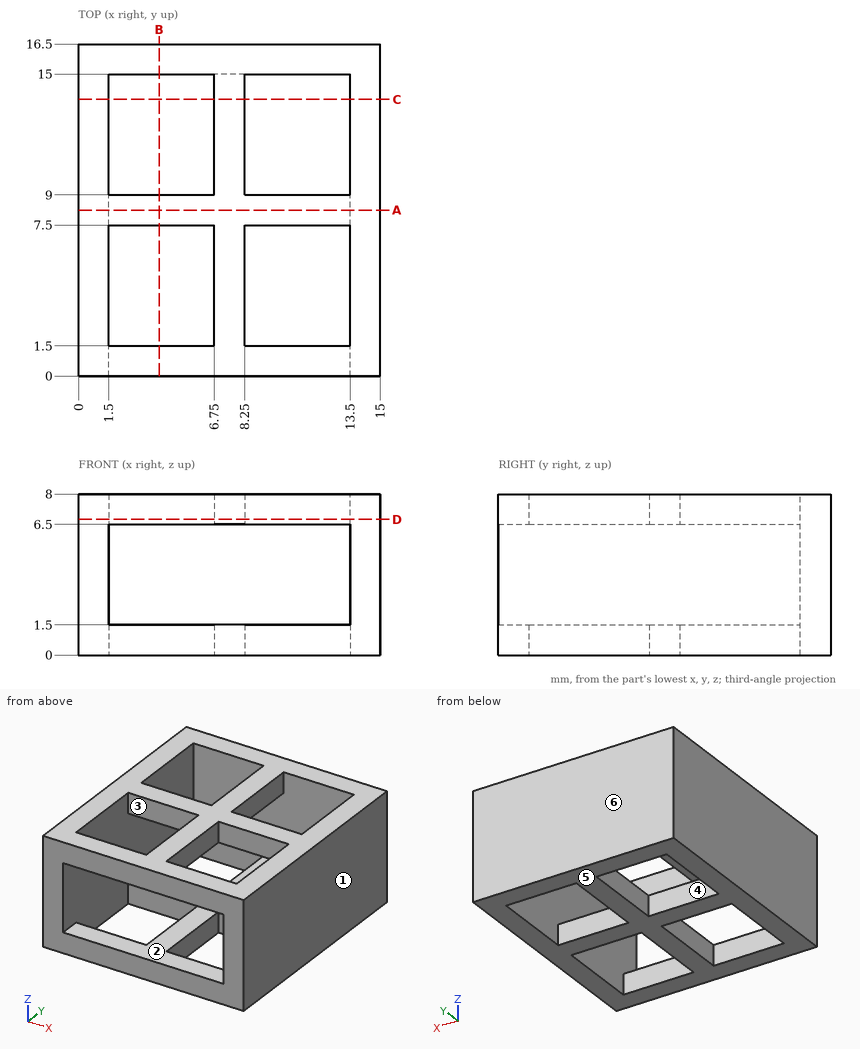
Input: dimensioned drawing with shaded views. Units: mm. Origin: part minimum x, y, z. A direction names the side the tool comes from. Coordinates: 2 decimals unless noted, no trailing zeros. Loops run counter-clockwise (first coordinate to the right, second up) from the corner with the lowest first, then second, coordinate; pieces in that order, holes last. Notation, with made-up numbers: M 63,34.25 L 80,34.25 A30 cw 80,59.25 Z; hole C 44,59 d6. An arc over 180 degrees is marked long. Use a Markdown table: item, result. Add a question column.
1) Section B-B, the plane x = 4. Return the cut outline in (y, z), plus the area to 3 significant figures.
2) Draft query along Y for the marked faces 4, 5 and 6. Return one class per face: +Y half, -Y half, draft (parallel to the pull), parting line (faces both ways), or undercut.
3) Section C-C, the plane y = 13.75. Return the cut outline in (x, z), plus the area to 3 significant figures.
4) Section A-A, the plane y = 8.25. Return the cut outline in (x, z), plus the area to 3 significant figures.
5) Section D-D, the plane z = 6.75. Return the cut outline in (x, y).
6) Line query: L1, parallel to Y at x = 4, z = 0.75; L2, parallel to X at y = 9.25, z = 7.75; L3, parallel to X at y = 9.5, z = 3.5. Output: solid intervals per line, ascending. Write a range as from..to.
7) Pin query (flat end, axial travel): P1, Ø1.2, axis at x = 4.5, z = 0.5, coming from the -Y side. Return the tip coordinate at first contact, or that it passes through.
8) Set-up query: the marked faces 1, 2 and 3. Return all of +Z, -Z, +X, -X, +Y, -Y with unobstructed straight access to the full face (end or side cutting, diameter ignored); none if empty.
Answer below:
| question | item | result |
|---|---|---|
| 1 | outline | M 0,0 L 1.5,0 L 1.5,1.5 L 0,1.5 Z; M 0,6.5 L 1.5,6.5 L 1.5,8 L 0,8 Z; M 7.5,0 L 9,0 L 9,1.5 L 7.5,1.5 Z; M 7.5,6.5 L 9,6.5 L 9,8 L 7.5,8 Z; M 15,0 L 16.5,0 L 16.5,8 L 15,8 Z |
| 1 | area | 21.0 mm2 |
| 2 | face 4 | undercut |
| 2 | face 5 | draft |
| 2 | face 6 | +Y half |
| 3 | outline | M 0,0 L 1.5,0 L 1.5,8 L 0,8 Z; M 6.75,0 L 8.25,0 L 8.25,1.5 L 6.75,1.5 Z; M 6.75,6.5 L 8.25,6.5 L 8.25,8 L 6.75,8 Z; M 13.5,0 L 15,0 L 15,8 L 13.5,8 Z |
| 3 | area | 28.5 mm2 |
| 4 | outline | M 0,0 L 15,0 L 15,8 L 0,8 Z; hole M 1.5,1.5 L 13.5,1.5 L 13.5,6.5 L 1.5,6.5 Z |
| 4 | area | 60.0 mm2 |
| 5 | outline | M 0,0 L 15,0 L 15,16.5 L 0,16.5 Z; hole M 1.5,1.5 L 6.75,1.5 L 6.75,7.5 L 1.5,7.5 Z; hole M 1.5,9 L 6.75,9 L 6.75,15 L 1.5,15 Z; hole M 8.25,1.5 L 13.5,1.5 L 13.5,7.5 L 8.25,7.5 Z; hole M 8.25,9 L 13.5,9 L 13.5,15 L 8.25,15 Z |
| 6 | L1 | 0..1.5, 7.5..9, 15..16.5 |
| 6 | L2 | 0..1.5, 6.75..8.25, 13.5..15 |
| 6 | L3 | 0..1.5, 13.5..15 |
| 7 | P1 | y = 0 |
| 8 | face 1 | +Z, -Z, +X, +Y, -Y |
| 8 | face 2 | -Y |
| 8 | face 3 | +Z, -Z |
